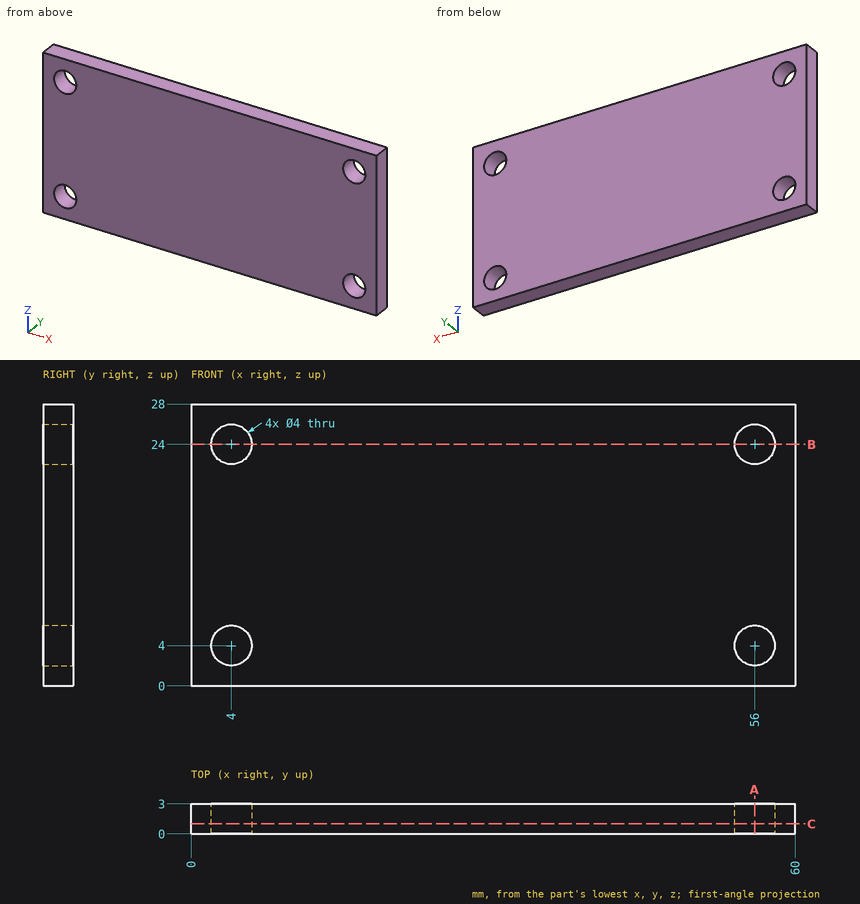
Can you work these out from the drawing? Everything is in mm from the part's minimum corner. Coordinates: 2 decimals unless noted, no trailing zeros. Write each loop counter-clockwise with the first axis right and the second up, starting at its lowest first coordinate (ties: lowest second). Pieces come first, ordered by that corner, then holes. Notation, with made-up numbers: (-32.5, 65.5) -> (14.5, 65.5) arc R14 cw to (14.5, 89.5) -> close; hole circle Ø8 at (-21.5, 15). An arc over 180 degrees is marked (long way). Write each question's results on one line, items separated by ' | '. Start each with the question number.
Q1. If I drill on probe 1 along Z at (x, y) = (56, 1.95); probe 2 along X at (y, z) = (2.3, 24); probe 3 along Z at (x, y) = (55, 2.7), over which ranges is the centre line in solid material (lowest first)?
Q2. I'm going to push a flat-ended pin straight in: pin 1 (3.5 mm diameter, centred on x = 4, z = 24, fed in from +Y). Where does the tip first touch, or does it pass through?
Q3. Imagine slicing it at C-C (y = 1). Write out the boundary of the cut face in (x, z).
Q4. Imagine slicing it at B-B (z = 24). Write out the boundary of the cut face in (x, y).
Q5. Imagine slicing it at A-A (x = 56). Write out the boundary of the cut face in (y, z), then the cut area to 3 significant figures.
Taken from the geometry:
1) probe 1: z = 0 to 2, 6 to 22, 26 to 28 | probe 2: x = 0 to 2, 6 to 54, 58 to 60 | probe 3: z = 0 to 2.27, 5.73 to 22.27, 25.73 to 28
2) pin 1: passes through
3) outline: (0, 0) -> (60, 0) -> (60, 28) -> (0, 28) -> close; hole circle Ø4 at (4, 4); hole circle Ø4 at (4, 24); hole circle Ø4 at (56, 4); hole circle Ø4 at (56, 24)
4) outline: (0, 0) -> (2, 0) -> (2, 3) -> (0, 3) -> close; (6, 0) -> (54, 0) -> (54, 3) -> (6, 3) -> close; (58, 0) -> (60, 0) -> (60, 3) -> (58, 3) -> close
5) outline: (0, 0) -> (3, 0) -> (3, 2) -> (0, 2) -> close; (0, 6) -> (3, 6) -> (3, 22) -> (0, 22) -> close; (0, 26) -> (3, 26) -> (3, 28) -> (0, 28) -> close | area: 60.0 mm^2
